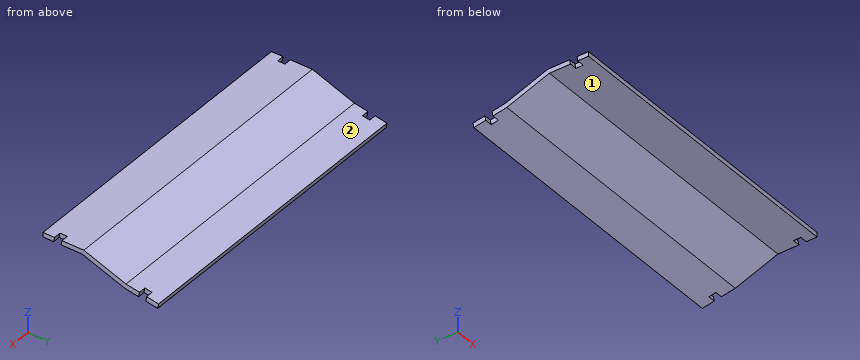
```python
from build123d import *

# Parameters (mm, degrees)
BOSS_EXTRUDE1_DEPTH = 322.072
CUT_EXTRUDE7_DEPTH  = 7.62
CUT_EXTRUDE8_DEPTH  = 7.62


with BuildPart() as part:
    # Sketch1 → Boss-Extrude1 (new body)
    with BuildSketch(Plane(origin=(0, 0, 0), x_dir=(0, 0, -1), z_dir=(1, 0, 0))):
        Polygon((222.810908306, 3.815774726), (227.813731692, 2.933641983), (221.740192501, -31.511110409), (205.541500449, -76.016651046), (205.541500449, -116.964716492), (200.767861936, -116.964716492), (200.767861936, -74.279188718), (216.814545731, -30.191287334), align=None)
    extrude(amount=BOSS_EXTRUDE1_DEPTH)

    # Sketch9 → Cut-Extrude7 (cut)
    with BuildSketch(Plane.ZY):
        Polygon((-228.475043657, -9.983148353), (-213.466573501, -7.336750125), (-212.143374387, -14.840985203), (-227.151844543, -17.487383431), align=None)
        Polygon((-209.00723387, -98.644141931), (-193.998763714, -95.997743703), (-193.998763714, -103.735294485), (-207.684034756, -106.148377008), align=None)
    extrude(amount=-CUT_EXTRUDE7_DEPTH, mode=Mode.SUBTRACT)

    # Sketch10 → Cut-Extrude8 (cut)
    with BuildSketch(Plane(origin=(322.072, 0, 0), x_dir=(0, 0, -1), z_dir=(1, 0, 0))):
        Polygon((228.475043657, -9.983148353), (213.466573501, -7.336750125), (212.143374387, -14.840985203), (227.151844543, -17.487383431), align=None)
        Polygon((193.998763714, -103.735294485), (207.684034756, -106.148377008), (209.00723387, -98.644141931), (193.998763714, -95.997743703), align=None)
    extrude(amount=-CUT_EXTRUDE8_DEPTH, mode=Mode.SUBTRACT)


solid = part.part
```
For this review, take the finished solid that the model builds, in its own axes (mm). Face numbers are marked on the shaded views. A direction names the side the tool comes from. Coordinates: 2 decimals unless noted, no trailing zeros. Write each loop counter-clockwise with the first axis right and the second up, starting at its lowest first coordinate (ties: lowest second). Pieces come first, ordered by that corner, then holes. Notation, with made-up numbers: (-24, -36) - (16, -36) arc R14 cw to (16, -26) - close; hole circle Ø3 at (-9, 14.25). An arc over 180 degrees is marked (long way). Put each result on its own line as item: value.
1. Add section A-A, the plane x = 171. Give the boundary of the cut face in (y, z), then the cut area to 3 significant figures.
Values found:
outline: (-116.96, -205.54) - (-76.02, -205.54) - (-31.51, -221.74) - (2.93, -227.81) - (3.82, -222.81) - (-30.19, -216.81) - (-74.28, -200.77) - (-116.96, -200.77) - close
area: 616 mm²
2. Machinability: for the marked faces 1 and 2, which of the approach directions +Z, -Z, +X, -X, +Y, -Y give a long, thin tool a straight path to every point of the face, cutting with its end or side? Answer none if there is none.
Values found:
face 1: -Z, +X, -X, -Y
face 2: +Z, +X, -X, +Y
3. Add section C-C, the plane z = -208.75. Give the boundary of the cut face in (x, y).
Values found:
outline: (0, -67.2) - (322.07, -67.2) - (322.07, -52.35) - (0, -52.35) - close
4. Add section B-B, the plane y = -84. Give the boundary of the cut face in (x, z), then the cut area to 3 significant figures.
Values found:
outline: (0, -205.54) - (322.07, -205.54) - (322.07, -200.77) - (0, -200.77) - close
area: 1,540 mm²
5. Wall thickness on probe 1 along X at (y, z) = (-104.5, -205.5); probe 2 along Z at (x, y) = (152, -106.5); probe 3 along Z at (x, y) = (239.5, -15): over which ranges is each line inside the solid? List them lowest first.
Values found:
probe 1: 7.62 to 314.45
probe 2: -205.54 to -200.77
probe 3: -224.65 to -219.49
6. For pin 1 (1.4 mm diameter, centred on y = -103.5, z = -202.5, fed in from +X); pin 2 (6 mm diameter, centred on x = 154, y = -102.5, fed in from -Z); pin 3 (1.5 mm diameter, centred on x = 86.5, y = -23.5, fed in from -Z) (3 decimals), all flat-tipped, find the tip position at first contact; note any pin that passes through.
Values found:
pin 1: x = 314.45
pin 2: z = -205.54
pin 3: z = -223.285
